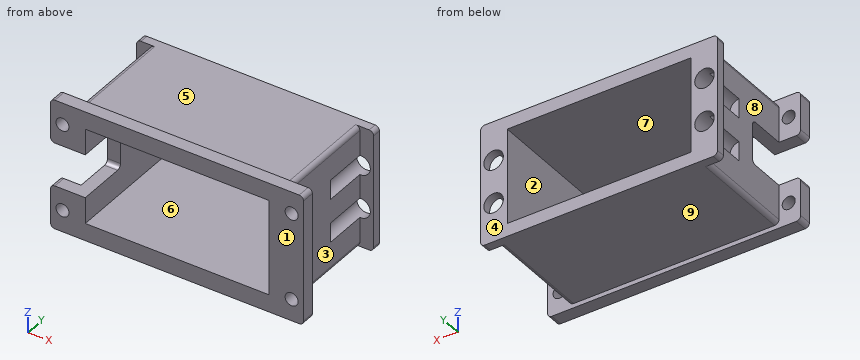
from build123d import *

# Parameters (mm, degrees)
SKETCH1_W           = 48.3
SKETCH1_H           = 28
SKETCH1_W_2         = 42.3
SKETCH1_H_2         = 22
BOSS_EXTRUDE1_DEPTH = 26.6
SKETCH2_W           = 54.6
SKETCH2_H           = 28
SKETCH2_W_2         = 42.3
SKETCH2_H_2         = 22
BOSS_EXTRUDE2_DEPTH = 2
SKETCH4_R           = 2.25
CUT_EXTRUDE1_DEPTH  = 12
SKETCH5_W           = 58.3
SKETCH5_H           = 30
SKETCH5_W_2         = 48.3
SKETCH5_H_2         = 28
BOSS_EXTRUDE3_DEPTH = 3
SKETCH6_W           = 10
SKETCH6_H           = 24
CUT_EXTRUDE2_DEPTH  = 10
SKETCH7_R           = 1.5
CUT_EXTRUDE3_DEPTH  = 10
FILLET1_R           = 1
FILLET2_R           = 1
FILLET3_R           = 1


with BuildPart() as part:
    # Sketch1 → Boss-Extrude1 (new body)
    with BuildSketch(Plane(origin=(0, 0, 0), x_dir=(1, 0, 0), z_dir=(0, 1, 0))):
        Rectangle(SKETCH1_W, SKETCH1_H)
        Rectangle(SKETCH1_W_2, SKETCH1_H_2, mode=Mode.SUBTRACT)
    extrude(amount=BOSS_EXTRUDE1_DEPTH)

    # Sketch2 → Boss-Extrude2 (add)
    with BuildSketch(Plane(origin=(0, 26.6, 0), x_dir=(1, 0, 0), z_dir=(0, 1, 0))):
        Rectangle(SKETCH2_W, SKETCH2_H)
        Rectangle(SKETCH2_W_2, SKETCH2_H_2, mode=Mode.SUBTRACT)
    extrude(amount=BOSS_EXTRUDE2_DEPTH)

    # Sketch4 → Cut-Extrude1 (cut)
    with BuildSketch(Plane(origin=(0, 28.6, 0), x_dir=(1, 0, 0), z_dir=(0, 1, 0))):
        with Locations(Location((-24.3, 5, 0), (0, 0, 270))):
            Circle(SKETCH4_R)
        with Locations(Location((-24.3, -5, 0), (0, 0, 270))):
            Circle(SKETCH4_R)
        with Locations(Location((24.3, 5, 0), (0, 0, 270))):
            Circle(SKETCH4_R)
        with Locations(Location((24.3, -5, 0), (0, 0, 270))):
            Circle(SKETCH4_R)
    extrude(amount=-CUT_EXTRUDE1_DEPTH, mode=Mode.SUBTRACT)

    # Sketch5 → Boss-Extrude3 (add)
    with BuildSketch(Plane.XZ):
        Rectangle(SKETCH5_W, SKETCH5_H)
        Rectangle(SKETCH5_W_2, SKETCH5_H_2, mode=Mode.SUBTRACT)
    extrude(amount=-BOSS_EXTRUDE3_DEPTH)

    # Sketch6 → Cut-Extrude2 (cut)
    with BuildSketch(Plane.ZY.offset(29.15)):
        Rectangle(SKETCH6_W, SKETCH6_H)
    extrude(amount=-CUT_EXTRUDE2_DEPTH, mode=Mode.SUBTRACT)

    # Sketch7 → Cut-Extrude3 (cut)
    with BuildSketch(Plane.XZ):
        with Locations(Location((-26.4, 10, 0), (0, 0, 270))):
            Circle(SKETCH7_R)
        with Locations(Location((-26.4, -10, 0), (0, 0, 270))):
            Circle(SKETCH7_R)
        with Locations(Location((26.4, 10, 0), (0, 0, 270))):
            Circle(SKETCH7_R)
        with Locations(Location((26.4, -10, 0), (0, 0, 270))):
            Circle(SKETCH7_R)
    extrude(amount=-CUT_EXTRUDE3_DEPTH, mode=Mode.SUBTRACT)

    # Fillet1
    fillet1_edges = [part.edges().sort_by_distance(p)[0] for p in [
        (-24.15, 14.8, -14),
        (24.15, 14.8, -14),
        (24.15, 14.8, 14),
        (-24.15, 14.8, 14),
    ]]
    fillet(fillet1_edges, radius=FILLET1_R)

    # Fillet2
    fillet2_edges = [part.edges().sort_by_distance(p)[0] for p in [
        (-29.15, 1.5, 5),
        (-29.15, 1.5, -5),
        (27.3, 27.6, 14),
        (27.3, 27.6, -14),
        (-27.3, 27.6, -14),
        (-27.3, 27.6, 14),
        (29.15, 1.5, 15),
        (29.15, 1.5, -15),
        (-29.15, 1.5, -15),
        (-29.15, 1.5, 15),
    ]]
    fillet(fillet2_edges, radius=FILLET2_R)

    # Fillet3
    fillet3_edges = [part.edges().sort_by_distance(p)[0] for p in [
        (-22.65, 12, -5),
        (-22.65, 12, 5),
    ]]
    fillet(fillet3_edges, radius=FILLET3_R)


solid = part.part
The model under review builds one solid part; all positions refer to its coordinate system, in mm. Face numbers are marked on the shaded views. A direction names the side the tool comes from. Coordinates: 2 decimals unless noted, no trailing zeros. Write each loop counter-clockwise with the first axis right and the second up, starting at its lowest first coordinate (ties: lowest second). Pieces come first, ordered by that corner, then holes. Notation, with made-up numbers: (-12, 56) -> (29, 56) arc R19 ccw to (29, 82) -> close; hole circle Ø4 at (31.25, 37). An arc over 180 degrees is marked (long way). Answer in a Markdown table with one row per item.
1. Wall thickness on probe 1 along X at (y, z) = (1.95, 10); probe 2 along X at (y, z) = (25.25, -5); probe 3 along Z at (x, y) = (15, 23.5): over which ranges is each line inside the solid? List them lowest first. Write a range as [from, to].
Answers below:
| item | result |
|---|---|
| probe 1 | x = [-29.15, -27.9], [-24.9, -21.15], [21.15, 24.9], [27.9, 29.15] |
| probe 2 | x = [-22.05, -21.15], [21.15, 22.05] |
| probe 3 | z = [-14, -11], [11, 14] |
2. We need section A-A, the plane y = 24.5. State the section outline as (x, z) points (3 decimals), and give its area (3 significant figures).
Answers below:
| item | result |
|---|---|
| outline | (-24.15, -13) arc R1 ccw to (-23.15, -14) -> (23.15, -14) arc R1 ccw to (24.15, -13) -> (24.15, -7.245) arc R2.25 cw to (24.15, -2.755) -> (24.15, 2.755) arc R2.25 cw to (24.15, 7.245) -> (24.15, 13) arc R1 ccw to (23.15, 14) -> (-23.15, 14) arc R1 ccw to (-24.15, 13) -> (-24.15, 7.245) arc R2.25 cw to (-24.15, 2.755) -> (-24.15, -2.755) arc R2.25 cw to (-24.15, -7.245) -> close; hole (-21.15, -11) -> (21.15, -11) -> (21.15, 11) -> (-21.15, 11) -> close |
| area | 392 mm^2 |
3. We need section D-D, the plane y = 15.75. State the section outline as (x, z) points, and give its area (3 significant figures).
Answers below:
| item | result |
|---|---|
| outline | (-24.15, -13) arc R1 ccw to (-23.15, -14) -> (23.15, -14) arc R1 ccw to (24.15, -13) -> (24.15, 13) arc R1 ccw to (23.15, 14) -> (-23.15, 14) arc R1 ccw to (-24.15, 13) -> close; hole (-21.15, -11) -> (21.15, -11) -> (21.15, 11) -> (-21.15, 11) -> close |
| area | 421 mm^2 |
4. For the marked faces 1, 2, 3, 4 and 5, list the 3-axis set-ups (+Z, -Z, +X, -X, +Y, -Y) from which the entire face can be reached by the end or side of a thin tool; tool diameter is ignored.
Answers below:
| item | result |
|---|---|
| face 1 | +Z, -Z, +X, -X, -Y |
| face 2 | +Y, -Y |
| face 3 | +Z, -Z, +X |
| face 4 | +Z, -Z, +X, -X, +Y |
| face 5 | +Z, +X, -X, +Y |
5. We need section B-B, the plane z = 10. State the section outline as (x, y) points.
Answers below:
| item | result |
|---|---|
| outline | (-29.15, 0) -> (-27.9, 0) -> (-27.9, 3) -> (-29.15, 3) -> close; (-27.3, 26.6) -> (-24.15, 26.6) -> (-24.15, 3) -> (-24.9, 3) -> (-24.9, 0) -> (-21.15, 0) -> (-21.15, 28.6) -> (-27.3, 28.6) -> close; (21.15, 0) -> (24.9, 0) -> (24.9, 3) -> (24.15, 3) -> (24.15, 26.6) -> (27.3, 26.6) -> (27.3, 28.6) -> (21.15, 28.6) -> close; (27.9, 0) -> (29.15, 0) -> (29.15, 3) -> (27.9, 3) -> close |
6. We need section C-C, the plane x = 15.5. State the section outline as (y, z) points, and give its area (3 significant figures).
Answers below:
| item | result |
|---|---|
| outline | (0, -15) -> (3, -15) -> (3, -14) -> (28.6, -14) -> (28.6, -11) -> (0, -11) -> close; (0, 11) -> (28.6, 11) -> (28.6, 14) -> (3, 14) -> (3, 15) -> (0, 15) -> close |
| area | 178 mm^2 |
7. Draft analysis for pull direction X (two halves, no side actions). For the marked faces 6, 7, 8 and 9, state which applies: +X half, -X half, draft (parallel to the pull), parting line (faces both ways), or undercut.
Answers below:
| item | result |
|---|---|
| face 6 | undercut |
| face 7 | undercut |
| face 8 | -X half |
| face 9 | draft |
8. Clearance check with flat-ended pins moving along their axes: pin 1 Ø5.5 at (x, y) = (-24.5, 6) entering from -Z; pin 2 Ø4 at (y, z) = (25.5, -7) entering from +X; pin 3 Ø2 at (y, z) = (27.5, 2.5) entering from -X; pin 4 Ø1.5 at (x, z) = (-8.5, -8.5) entering from +Y. State where each tip first meets the part, or that it passes through.
Answers below:
| item | result |
|---|---|
| pin 1 | stops at z = -14 |
| pin 2 | stops at x = 27.3 |
| pin 3 | stops at x = -27.3 |
| pin 4 | passes through |
